The model under review builds one solid part; all positions refer to its coordinate system, in mm. Face numbers are marked on the shaded views. A direction names the side the tool comes from. Coordinates: 2 decimals unless noted, no trailing zeros. Order: outer loops, then holes, each group sorted by start corner. A loop starts at its lowest first (then second) coordinate and runs counter-clockwise, first axis right, second up. Notation, with made-up numbers: M -36,-7 L -2,-7 A29 ccw -2,30 Z; hole C 46.5,43.5 d1. An arc over 180 degrees is marked long. Answer in a Markdown table with one row per item.
from build123d import *

# Parameters (mm, degrees)
SKETCH_1_R          = 5
EXTRUDE_1_DEPTH     = 4
SKETCH_2_R          = 12
EXTRUDE_2_DEPTH     = 2
EXTRUDE_START       = 2
SKETCH_3_R          = 12
EXTRUDE_3_DEPTH     = 2
EXTRUDE_START_2     = 6
SKETCH_4_R          = 5
EXTRUDE_4_DEPTH     = 6
SKETCH_5_R          = 2
CUT_EXTRUDE_1_DEPTH = 23
FILLET_2_R          = 1


with BuildPart() as part:
    # 草图1 → 凸台-拉伸1 (new body)
    with BuildSketch(Plane(origin=(0, 0, 0), x_dir=(1, 0, 0), z_dir=(0, 1, 0))):
        with Locations(Location((0, 0, 0), (0, 0, 270))):
            Circle(SKETCH_1_R)
    extrude(amount=EXTRUDE_1_DEPTH)

    # 草图2 → 凸台-拉伸2 (add)
    with BuildSketch(Plane(origin=(0, 4, 0), x_dir=(1, 0, 0), z_dir=(0, 1, 0))):
        with Locations(Location((0, 0, 0), (0, 0, 270))):
            Circle(SKETCH_2_R)
    extrude(amount=EXTRUDE_2_DEPTH)

    # 草图3 → 凸台-拉伸3 (add)
    with BuildSketch(Plane.XZ.offset(EXTRUDE_START)):
        with Locations(Location((0, 0, 0), (0, 0, 90))):
            Circle(SKETCH_3_R)
    extrude(amount=-EXTRUDE_3_DEPTH)

    # 草图4 → 凸台-拉伸4 (add)
    with BuildSketch(Plane(origin=(0, -2, 0), x_dir=(-1, 0, 0), z_dir=(0, -1, 0)).offset(EXTRUDE_START_2)):
        with Locations(Location((0, 0, 0), (0, 0, 270))):
            Circle(SKETCH_4_R)
    extrude(amount=-EXTRUDE_4_DEPTH)

    # 草图5 → 切除-拉伸1 (cut, through all)
    with BuildSketch(Plane.XZ.offset(8)):
        with Locations(Location((0, 0, 0), (0, 0, 270))):
            Circle(SKETCH_5_R)
    extrude(amount=-CUT_EXTRUDE_1_DEPTH, mode=Mode.SUBTRACT)

    # 圆角2
    fillet_2_edges = [part.edges().sort_by_distance(p)[0] for p in [
        (0, -2, -12),
        (0, 4, -12),
        (0, 6, -12),
        (0, 0, -12),
    ]]
    fillet(fillet_2_edges, radius=FILLET_2_R - 0.0001)  # a hair under: the kernel refuses the full size


solid = part.part
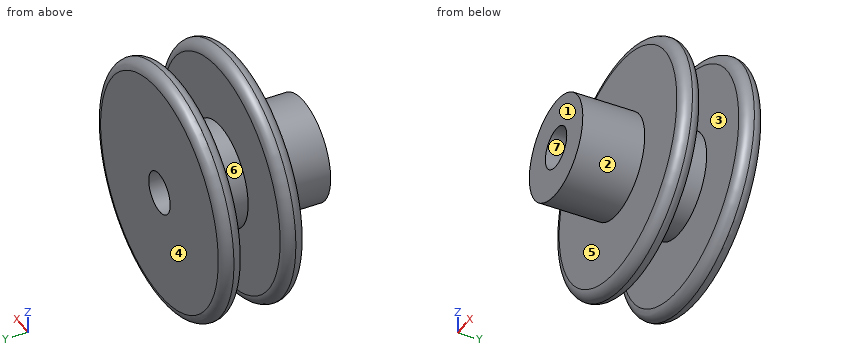
(1) To check wall thickness, follow line 1 (Y direction, x = -5, z = 9.75); line 2 (X direction, y = -3.25, z = 0); line 3 (X direction, y = 3, z = -0.75). State the ranges of each line that lie inside material, in increasing order. Write a range as [from, to].
Report:
| item | result |
|---|---|
| line 1 | [-2, 0], [4, 6] |
| line 2 | [-5, -2], [2, 5] |
| line 3 | [-4.94, -1.85], [1.85, 4.94] |
(2) Machinability: for the marked faces 1, 2 and 3, which of the approach directions +Z, -Z, +X, -X, +Y, -Y give a long, thin tool a straight path to every point of the face, cutting with its end or side? Answer none if there is none.
Report:
| item | result |
|---|---|
| face 1 | +Z, -Z, +X, -X, -Y |
| face 2 | -Y |
| face 3 | none |
(3) Take a section at C-C (y = -6.75). Write out the cut boundary in (x, z).
Report:
| item | result |
|---|---|
| outline | C 0,0 d10; hole C 0,0 d4 |
(4) Insertion check: P1, Ø8, axis at y = -1, z = 3, coming from the +X side; P2, Ø2, axis at y = 2.5, z = 3, coming from the -X side; P3, Ø2, axis at x = 7, z = -8.5, coming from the -Y side; P4, Ø4, axis at y = -3.5, z = 2.5, coming from the +X side. Each pin has a flat end and moves straight along its axis. Give the tip position at first contact, or say it passes through.
Report:
| item | result |
|---|---|
| P1 | x = 12 |
| P2 | x = -4.58 |
| P3 | y = -2 |
| P4 | x = 11.66 |
(5) The part is to be moulded in two halves that separate along Y. For the marked faces 4, 5, 6 and 7, say which applies: +Y half, -Y half, draft (parallel to the pull), parting line (faces both ways), or undercut.
Report:
| item | result |
|---|---|
| face 4 | +Y half |
| face 5 | -Y half |
| face 6 | undercut |
| face 7 | draft |
(6) Take a section at D-D (y = -0.5). Write out the cut boundary in (x, z).
Report:
| item | result |
|---|---|
| outline | C 0,0 d23.73; hole C 0,0 d4 |
